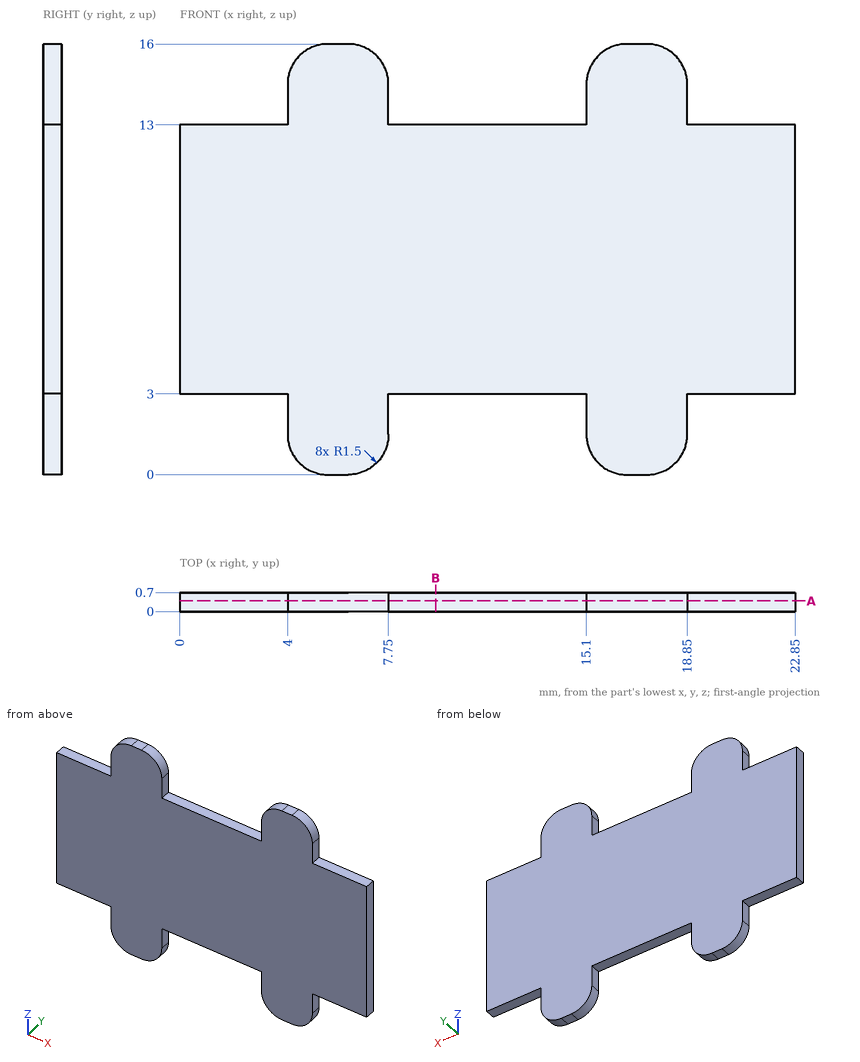
Study the drawing (mm; zero at the part's minimum x, y, z) and answer. Give positions to 0.01 mm unless a question says otherwise; leave off trailing zeros. Order: outer loops, then holes, each group sorted by start corner. A loop starts at its lowest first (then second) coordinate and runs counter-clockwise, first axis right, second up. Notation, with made-up numbers: M 73,37 L 111,37 A17 cw 111,67 Z; hole C 68,29 d7. An arc over 180 degrees is marked long. Put each result on its own line as item: value. Start each with the question number.
Item 1: The part is cut by section B-B, the plane x = 9.5. Determine the outline of the cut face in (y, z).
Item 2: The part is cut by section A-A, the plane y = 0.4. Determine the outline of the cut face in (x, z).
Item 3: A flat-ended cylindrical pin translates along its axis: P1, Ø8, axis at x = 4.5, z = 14, coming from the -Y side. Find the tip coordinate at first contact, or state that the pin passes through.
Item 4: Find the intervals of material crossed by line 1 along X through (y, z) = (0.35, 13.25); line 2 along Z through (x, y) = (21, 0.15); line 3 along X through (y, z) = (0.3, 1), in increasing order.
Answer key:
1. outline: M 0,3 L 0.7,3 L 0.7,13 L 0,13 Z
2. outline: M 0,3 L 4,3 L 4,1.5 A1.5 ccw 5.5,0 L 6.25,0 A1.5 ccw 7.75,1.5 L 7.75,3 L 15.1,3 L 15.1,1.5 A1.5 ccw 16.6,0 L 17.35,0 A1.5 ccw 18.85,1.5 L 18.85,3 L 22.85,3 L 22.85,13 L 18.85,13 L 18.85,14.5 A1.5 ccw 17.35,16 L 16.6,16 A1.5 ccw 15.1,14.5 L 15.1,13 L 7.75,13 L 7.75,14.5 A1.5 ccw 6.25,16 L 5.5,16 A1.5 ccw 4,14.5 L 4,13 L 0,13 Z
3. P1: stops at y = 0
4. line 1: x = 4 to 7.75, 15.1 to 18.85
4. line 2: z = 3 to 13
4. line 3: x = 4.09 to 7.66, 15.19 to 18.76
